```python
from build123d import *

# Parameters (mm, degrees)
EXTRUDE_1_DEPTH = 2


with BuildPart() as part:
    # 草图1 → 凸台-拉伸1 (new body)
    with BuildSketch(Plane.XY):
        with BuildLine():
            Line((32.521472611, 127.716716237), (26.282107631, 127.716716237))
            Line((26.282107631, 127.716716237), (26.282107631, 126.216716237))
            Line((26.282107631, 126.216716237), (21.740638301, 126.216716237))
            ThreePointArc((21.740638301, 126.216716237), (24.74234251, 124.860533901), (25.708617606, 121.711602158))
            Line((25.708617606, 121.711602158), (22.586955956, 97.189045118))
            ThreePointArc((22.586955956, 97.189045118), (20.600713495, 93.444159924), (16.634986998, 91.946716237))
            Line((16.634986998, 91.946716237), (21.919620287, 91.946716237))
            Line((21.919620287, 91.946716237), (21.919620287, 90.446716237))
            Line((21.919620287, 90.446716237), (17.187204618, 90.446716237))
            ThreePointArc((17.187204618, 90.446716237), (20.188908827, 89.090533901), (21.155183923, 85.941602158))
            Line((21.155183923, 85.941602158), (11.419141111, 9.459045118))
            ThreePointArc((11.419141111, 9.459045118), (9.43289865, 5.714159924), (5.467172154, 4.216716237))
            Line((5.467172154, 4.216716237), (10.751805442, 4.216716237))
            Line((10.751805442, 4.216716237), (10.751805442, 2.716716237))
            Line((10.751805442, 2.716716237), (16.609277745, 2.716716237))
            Line((16.609277745, 2.716716237), (32.521472611, 127.716716237))
        make_face()
    extrude(amount=EXTRUDE_1_DEPTH)


solid = part.part
```
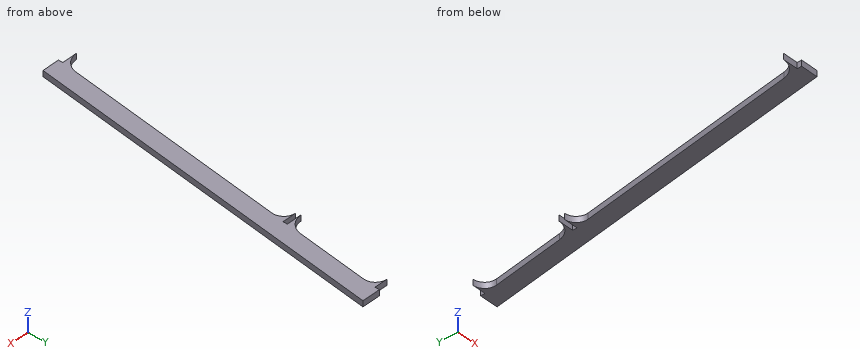
Input: part model. Units: mm. Frame: model coordinates. Round coordinates to 2 decimals unless told otherwise and drop trailing zeros. Write each loop counter-clockwise with the first axis right and the second up, starting at its lowest first coordinate (ties: lowest second). Pieces come first, ordered by that corner, then holes. Notation, with made-up numbers: (48.25, 87) - (77.25, 87) arc R13 ccw to (77.25, 104) - close; hole circle Ø5 at (53, -32). An arc over 180 degrees is marked (long way). Write item = value, one per line.
(1) Material intervals for probe 1 along X at (y, z) = (50, 1.6); probe 2 along X at (y, z) = (13, 1.8); probe 3 along Y at (x, z) = (7, 0.55), sorted ascending.
Geometry check:
probe_1 = 16.58 to 22.63
probe_2 = 11.87 to 17.92
probe_3 = 4.22 to 4.42
(2) Section query B-B on x = 19. Output: boundary loops of the cut face in (y, z).
Geometry check:
outline = (21.5, 0) - (69.01, 0) - (69.01, 2) - (21.5, 2) - close; (90.01, 0) - (90.45, 0) - (90.45, 2) - (90.01, 2) - close; (91.95, 0) - (92.43, 0) - (92.43, 2) - (91.95, 2) - close
(3) Contact query for flat-ended pins moving along their axis: pin 1 Ø1 at (x, z) = (20, 0.5) entering from +Y; pin 2 Ø1 at (x, z) = (10, 0.5) entering from +Y; pin 3 Ø0.8 at (y, z) = (91.5, 0.5) entering from -X. Output: stop coordinate, or through.
Geometry check:
pin_1 = 93.36
pin_2 = 6.95
pin_3 = 21.92
(4) Section query D-D on x = 14. Output: boundary loops of the cut face in (y, z).
Geometry check:
outline = (2.72, 0) - (29.73, 0) - (29.73, 2) - (2.72, 2) - close
(5) Section query A-A on z = 0.75. Output: boundary loops of the cut face in (x, y).
Geometry check:
outline = (5.47, 4.22) - (10.75, 4.22) - (10.75, 2.72) - (16.61, 2.72) - (32.52, 127.72) - (26.28, 127.72) - (26.28, 126.22) - (21.74, 126.22) arc R4 cw to (25.71, 121.71) - (22.59, 97.19) arc R6 cw to (16.63, 91.95) - (21.92, 91.95) - (21.92, 90.45) - (17.19, 90.45) arc R4 cw to (21.16, 85.94) - (11.42, 9.46) arc R6 cw to start
(6) Section query C-C on y = 81. Output: boundary loops of the cut face in (x, z).
Geometry check:
outline = (20.53, 0) - (26.57, 0) - (26.57, 2) - (20.53, 2) - close
